Read the model definition and answer for the solid it produces. Units are mm, in the model's axes. Face numbers are marked on the shaded views. A direction names the side the tool comes from. Coordinates: 2 decimals unless noted, no trailing zeros. Order: outer loops, then holes, each group sorted by start corner. A loop starts at its lowest first (then second) coordinate and runs counter-clockwise, first axis right, second up. Notation, with made-up numbers: (45.5, 27) -> (62.5, 27) arc R16 ccw to (62.5, 40) -> close; hole circle Ø2 at (5.5, 61.25). An arc over 180 degrees is marked (long way). Answer as a JSON object with one key per item and string values. Group by question number.
1) Determine the mould class of the marked faces 5, 6, 7 and 8 for opening direction X: released by +X, released by -X, zero draft, split by the parting line, or undercut.
2) Consider L1, parallel to X at y = 5.25, z = -7; L2, parallel to X at y = 0.6, z = -7; L3, parallel to X at y = 0.95, z = -7. Determine where each line is inside the solid, lowest interval first.
3) Section C-C on y = 4.25 is taken. Determine the outline of the cut face in (x, z), and give its area (3 significant figures).
4) Given pin 1 (6 mm diameter, centred on x = -4.5, z = -3.5, fed in from +Y); pin 2 (6.5 mm diameter, centred on x = 15.5, z = -7.5, fed in from +Y); pin 3 (5 mm diameter, centred on x = 1.5, z = -7.5, fed in from +Y); pin 4 (3.5 mm diameter, centred on x = -13, z = -7, fed in from +Y), each flat-ended and moving along its own axis, determine where each tip first touches the part or whether it passes through.
5) A tool of negligible diameter and unlimited length cuts with its end or side. For the marked faces 1, 2, 3 and 4, from which of +Z, -Z, +X, -X, +Y, -Y can it reach the whole face along a straight path? Write none if from no direction.
6) Section A-A on z = -7 is taken. Determine the outline of the cut face in (x, y).
7) Section D-D on x = -12.5 is taken. Determine the outline of the cut face in (y, z), and give its area (3 significant figures).
8) Section B-B on x = 12 is taken. Determine the outline of the cut face in (y, z), and give its area (3 significant figures).
from build123d import *

# Parameters (mm, degrees)
BOSS_EXTRUDE1_DEPTH = 7
SKETCH2_R           = 2.75
CUT_EXTRUDE1_DEPTH  = 26.396850198
SKETCH3_R           = 5
CUT_EXTRUDE2_DEPTH  = 4
SKETCH4_R           = 5.25
CUT_EXTRUDE3_DEPTH  = 26.396850198
BOSS_EXTRUDE2_DEPTH = 14


with BuildPart() as part:
    # Sketch1 → Boss-Extrude1 (new body)
    with BuildSketch(Plane(origin=(0, 0, 0), x_dir=(1, 0, 0), z_dir=(0, 1, 0))):
        with BuildLine():
            Line((-13, 0), (13, 0))
            ThreePointArc((13, 0), (20, 7), (13, 14))
            Line((13, 14), (-13, 14))
            ThreePointArc((-13, 14), (-20, 7), (-13, 0))
        make_face()
    extrude(amount=BOSS_EXTRUDE1_DEPTH)

    # Sketch2 → Cut-Extrude1 (cut, through all)
    with BuildSketch(Plane(origin=(0, 7, 0), x_dir=(1, 0, 0), z_dir=(0, 1, 0))):
        with Locations(Location((-13, 7, 0), (0, 0, 270))):
            Circle(SKETCH2_R)
        with Locations(Location((13, 7, 0), (0, 0, 90))):
            Circle(SKETCH2_R)
    extrude(amount=-CUT_EXTRUDE1_DEPTH, mode=Mode.SUBTRACT)

    # Sketch3 → Cut-Extrude2 (cut)
    with BuildSketch(Plane(origin=(0, 7, 0), x_dir=(1, 0, 0), z_dir=(0, 1, 0))):
        with Locations(Location((-13, 7, 0), (0, 0, 270))):
            Circle(SKETCH3_R)
        with Locations(Location((13, 7, 0), (0, 0, 90))):
            Circle(SKETCH3_R)
    extrude(amount=-CUT_EXTRUDE2_DEPTH, mode=Mode.SUBTRACT)

    # Sketch4 → Cut-Extrude3 (cut, through all)
    with BuildSketch(Plane.XY):
        with Locations((0, -0.5)):
            Circle(SKETCH4_R)
    extrude(amount=-CUT_EXTRUDE3_DEPTH, mode=Mode.SUBTRACT)

    # Sketch5 → Boss-Extrude2 (add)
    with BuildSketch(Plane.XY):
        with BuildLine():
            Line((-6.614378278, 7), (6.614378278, 7))
            ThreePointArc((6.614378278, 7), (0, 9.5), (-6.614378278, 7))
        make_face()
    extrude(amount=-BOSS_EXTRUDE2_DEPTH)


solid = part.part
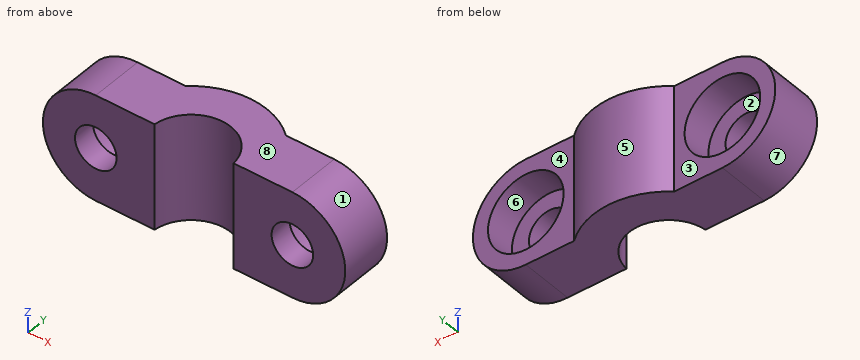
Worked answers:
{
 "1": {"face 5": "split by the parting line", "face 6": "undercut", "face 7": "released by -X", "face 8": "zero draft"},
 "2": {"L1": "x = -20 to -18, -8 to 8, 18 to 20", "L2": "x = -20 to -15.75, -10.25 to -5.13, 5.13 to 10.25, 15.75 to 20", "L3": "x = -20 to -15.75, -10.25 to -5.05, 5.05 to 10.25, 15.75 to 20"},
 "3": {"outline": "(-13, -14) -> (-2.24, -14) -> (-2.24, 0) -> (-13, 0) arc R7 ccw to start; (2.24, -14) -> (13, -14) arc R7 ccw to (13, 0) -> (2.24, 0) -> close; hole circle Ø10 at (-13, -7); hole circle Ø10 at (13, -7)", "area": "298 mm²"},
 "4": {"pin 1": "stops at y = 9.39", "pin 2": "stops at y = 7", "pin 3": "stops at y = 9.5", "pin 4": "passes through"},
 "5": {"face 1": "+X, +Y, -Y", "face 2": "+Y", "face 3": "+Z, -Z, -X, +Y", "face 4": "+Z, -Z, +X, +Y"},
 "6": {"outline": "(-20, 0) -> (-15.75, 0) -> (-15.75, 3) -> (-18, 3) -> (-18, 7) -> (-20, 7) -> close; (-10.25, 0) -> (-5.23, 0) arc R5.25 cw to (5.23, 0) -> (10.25, 0) -> (10.25, 3) -> (8, 3) -> (8, 7) -> (6.61, 7) arc R10 ccw to (-6.61, 7) -> (-8, 7) -> (-8, 3) -> (-10.25, 3) -> close; (15.75, 0) -> (20, 0) -> (20, 7) -> (18, 7) -> (18, 3) -> (15.75, 3) -> close"},
 "7": {"outline": "(0, -14) -> (7, -14) -> (7, -11.97) -> (3, -11.97) -> (3, -9.7) -> (0, -9.7) -> close; (0, -4.3) -> (3, -4.3) -> (3, -2.03) -> (7, -2.03) -> (7, 0) -> (0, 0) -> close", "area": "42.0 mm²"},
 "8": {"outline": "(0, -14) -> (7, -14) -> (7, -11.9) -> (3, -11.9) -> (3, -9.56) -> (0, -9.56) -> close; (0, -4.44) -> (3, -4.44) -> (3, -2.1) -> (7, -2.1) -> (7, 0) -> (0, 0) -> close", "area": "43.4 mm²"}
}
